from build123d import *

# Parameters (mm, degrees)
SKETCH3_R                              = 50
BOSS_EXTRUDE1_DEPTH                    = 10
SKETCH4_R                              = 20
CUT_EXTRUDE3_DEPTH                     = 10
BOSS_EXTRUDE3_DEPTH                    = 50
CBORE_FOR_M6_HEX_HEAD_BOLT1_AT_2_COUNT = 2
CBORE_FOR_M6_HEX_HEAD_BOLT1_AT_2_PITCH = 70
CBORE_FOR_M6_HEX_HEAD_BOLT4_AT_2_COUNT = 2
CBORE_FOR_M6_HEX_HEAD_BOLT4_AT_2_PITCH = 70


with BuildPart() as part:
    # Sketch3 → Boss-Extrude1 (new body)
    with BuildSketch(Plane(origin=(0, 0, 0), x_dir=(1, 0, 0), z_dir=(0, 1, 0))):
        Circle(SKETCH3_R)
    extrude(amount=BOSS_EXTRUDE1_DEPTH)

    # Sketch4 → Cut-Extrude3 (cut)
    with BuildSketch(Plane(origin=(0, 10, 0), x_dir=(1, 0, 0), z_dir=(0, 1, 0))):
        Circle(SKETCH4_R)
    extrude(amount=-CUT_EXTRUDE3_DEPTH, mode=Mode.SUBTRACT)

    # Sketch5 → Boss-Extrude3 (add)
    with BuildSketch(Plane(origin=(0, 10, 0), x_dir=(1, 0, 0), z_dir=(0, 1, 0))):
        with BuildLine():
            ThreePointArc((14.142135624, 14.142135624), (20, 0), (14.142135624, -14.142135624))
            Line((14.142135624, -14.142135624), (35.355339059, -35.355339059))
            ThreePointArc((35.355339059, -35.355339059), (50, 0), (35.355339059, 35.355339059))
            Line((35.355339059, 35.355339059), (14.142135624, 14.142135624))
        make_face()
        with BuildLine():
            ThreePointArc((-14.142135624, -14.142135624), (-20, 0), (-14.142135624, 14.142135624))
            Line((-14.142135624, 14.142135624), (-35.355339059, 35.355339059))
            ThreePointArc((-35.355339059, 35.355339059), (-50, 0), (-35.355339059, -35.355339059))
            Line((-35.355339059, -35.355339059), (-14.142135624, -14.142135624))
        make_face()
    extrude(amount=BOSS_EXTRUDE3_DEPTH)

    # Sketch7 → CBORE for M6 Hex Head Bolt1 (revolve, cut)
    with BuildSketch(Plane(origin=(-35, 60, 0), x_dir=(0, 0, 1), z_dir=(1, 0, 0))):
        Polygon((0, 0), (0, 60), (3.38, 60), (3.38, 4.19), (7.145, 4.19), (7.145, 0.635), (7.78, 0), align=None)
    cbore_for_m6_hex_head_bolt1 = revolve(axis=Axis((-35, 66.35, 0), (0, -1, 0)), mode=Mode.SUBTRACT)

    # CBORE for M6 Hex Head Bolt1 at 2: CBORE for M6 Hex Head Bolt1 ×2
    with Locations(*[(i * CBORE_FOR_M6_HEX_HEAD_BOLT1_AT_2_PITCH, 0, 0) for i in range(1, CBORE_FOR_M6_HEX_HEAD_BOLT1_AT_2_COUNT)]):
        add(cbore_for_m6_hex_head_bolt1, mode=Mode.SUBTRACT)

    # Sketch17 → CBORE for M6 Hex Head Bolt4 (revolve, cut)
    with BuildSketch(Plane(origin=(0, 10, -35), x_dir=(0, 0, 1), z_dir=(1, 0, 0))):
        Polygon((0, 0), (0, 10), (3.38, 10), (3.38, 4.19), (7.145, 4.19), (7.145, 0.635), (7.78, 0), align=None)
    cbore_for_m6_hex_head_bolt4 = revolve(axis=Axis((0, 16.35, -35), (0, -1, 0)), mode=Mode.SUBTRACT)

    # CBORE for M6 Hex Head Bolt4 at 2: CBORE for M6 Hex Head Bolt4 ×2
    with Locations(*[(0, 0, i * CBORE_FOR_M6_HEX_HEAD_BOLT4_AT_2_PITCH) for i in range(1, CBORE_FOR_M6_HEX_HEAD_BOLT4_AT_2_COUNT)]):
        add(cbore_for_m6_hex_head_bolt4, mode=Mode.SUBTRACT)


solid = part.part
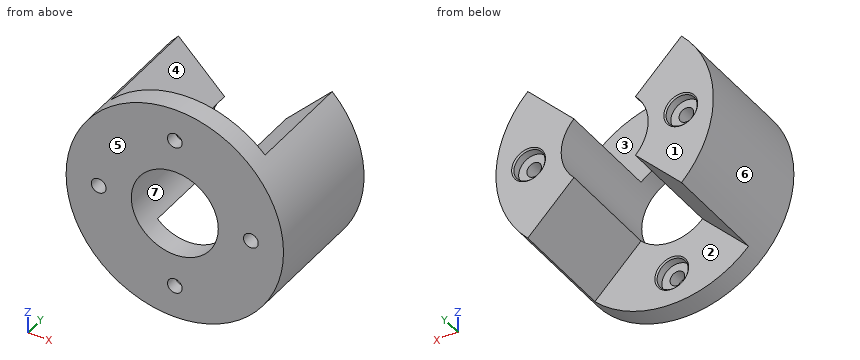
Geometry: final body of the model. Coordinates: model frame, mm. Face numbers are marked on the shaded views. A direction names the side the tool comes from. Coordinates: 2 decimals unless noted, no trailing zeros. Write each loop counter-clockwise with the first axis right and the second up, starting at its lowest first coordinate (ties: lowest second). Pieces come first, ordered by that corner, then holes. Notation, with made-up numbers: (65.5, -8) - (107.5, -8) arc R27 cw to (107.5, 8) - close; hole circle Ø1 at (-22, 53.5). An arc over 180 degrees is marked (long way). Return JSON: item names as keys, results as strings.
Item 1: Section query A-A (x = 0). Output: boundary loops of the cut face in (y, z) (3 decimals), and give its area (3 significant figures).
Completed:
{"outline": "(0, -50) - (10, -50) - (10, -42.78) - (9.365, -42.145) - (5.81, -42.145) - (5.81, -38.38) - (0, -38.38) - close; (0, -31.62) - (5.81, -31.62) - (5.81, -27.855) - (9.365, -27.855) - (10, -27.22) - (10, -20) - (0, -20) - close; (0, 20) - (10, 20) - (10, 27.22) - (9.365, 27.855) - (5.81, 27.855) - (5.81, 31.62) - (0, 31.62) - close; (0, 38.38) - (5.81, 38.38) - (5.81, 42.145) - (9.365, 42.145) - (10, 42.78) - (10, 50) - (0, 50) - close", "area": "401 mm2"}
Item 2: Pull-direction query (Z, two-part tool) for the marked faces 4, 5, 6 and 7; classes: +Z half, -Z half, draft (parallel to the pull), parting line (faces both ways), or undercut.
Completed:
{"face 4": "+Z half", "face 5": "draft", "face 6": "parting line", "face 7": "undercut"}
Item 3: Pin query (flat end, axial travel): pin 1 Ø1.5 at (y, z) = (11, 21) entering from +X; pin 2 Ø6 at (y, z) = (6.5, -6) entering from -X; pin 3 Ø1.5 at (y, z) = (43, 24) entering from -X. Return the tip coordinate at first contact, or that it passes through.
Completed:
{"pin 1": "stops at x = 45.72", "pin 2": "stops at x = -49.91", "pin 3": "stops at x = -44.27"}
Item 4: Line query: L1, parallel to X at y = 57, z = 0 (3 decimals); L2, parallel to Z at x = 0, y = 3.8. Output: solid intervals per line, ascending.
Completed:
{"L1": "x = -50 to -42.145, -27.855 to -20, 20 to 27.855, 42.145 to 50", "L2": "z = -50 to -38.38, -31.62 to -20, 20 to 31.62, 38.38 to 50"}
Item 5: Reachability of the marked faces 1, 2 and 3 from +Z, -Z, +X, -X, +Y, -Y: full face, straight path, thin tool, end or side. Return the list, or none.
Completed:
{"face 1": "+Z, -Z, +X, -X, +Y", "face 2": "-Z, +Y", "face 3": "+Z, +Y"}
